Here's how the part is built. I have some questions about the finished solid (model axes, mm). Round coordinates to 2 decimals unless told otherwise and drop trailing zeros. Write each loop counter-clockwise with the first axis right and the second up, starting at its lowest first coordinate (ties: lowest second). Pieces come first, ordered by that corner, then holes. Notation, with made-up numbers: (38, -25.75) -> (79, -25.75) arc R34 ccw to (79, 11.25) -> close; hole circle Ø3 at (-18, 40.25). An arc over 180 degrees is marked (long way). Answer in a Markdown table with one row per item.
from build123d import *

# Parameters (mm, degrees)
SKETCH1_W           = 234.95
SKETCH1_H           = 228.6
BOSS_EXTRUDE1_DEPTH = 50.8
SKETCH2_R           = 4.826
CUT_EXTRUDE1_DEPTH  = 38.1
SKETCH3_R           = 6.477
CUT_EXTRUDE2_DEPTH  = 38.1


with BuildPart() as part:
    # Sketch1 → Boss-Extrude1 (new body)
    with BuildSketch(Plane(origin=(0, 0, 0), x_dir=(1, 0, 0), z_dir=(0, 1, 0))):
        with Locations((117.475, 114.3)):
            Rectangle(SKETCH1_W, SKETCH1_H)
    extrude(amount=BOSS_EXTRUDE1_DEPTH)

    # Sketch2 → Cut-Extrude1 (cut)
    with BuildSketch(Plane(origin=(0, 50.8, 0), x_dir=(1, 0, 0), z_dir=(0, 1, 0))):
        with Locations(Location((74.549, 170.307, 0), (0, 0, 270))):
            Circle(SKETCH2_R)
        with Locations(Location((160.401, 170.307, 0), (0, 0, 270))):
            Circle(SKETCH2_R)
        with Locations(Location((160.401, 58.293, 0), (0, 0, 270))):
            Circle(SKETCH2_R)
        with Locations(Location((74.549, 58.293, 0), (0, 0, 270))):
            Circle(SKETCH2_R)
    extrude(amount=-CUT_EXTRUDE1_DEPTH, mode=Mode.SUBTRACT)

    # Sketch3 → Cut-Extrude2 (cut)
    with BuildSketch(Plane(origin=(0, 50.8, 0), x_dir=(1, 0, 0), z_dir=(0, 1, 0))):
        with Locations(Location((196.85, 153.67, 0), (0, 0, 270))):
            Circle(SKETCH3_R)
        with Locations(Location((196.85, 74.93, 0), (0, 0, 270))):
            Circle(SKETCH3_R)
        with Locations(Location((38.1, 74.93, 0), (0, 0, 270))):
            Circle(SKETCH3_R)
        with Locations(Location((38.1, 153.67, 0), (0, 0, 270))):
            Circle(SKETCH3_R)
    extrude(amount=-CUT_EXTRUDE2_DEPTH, mode=Mode.SUBTRACT)


solid = part.part
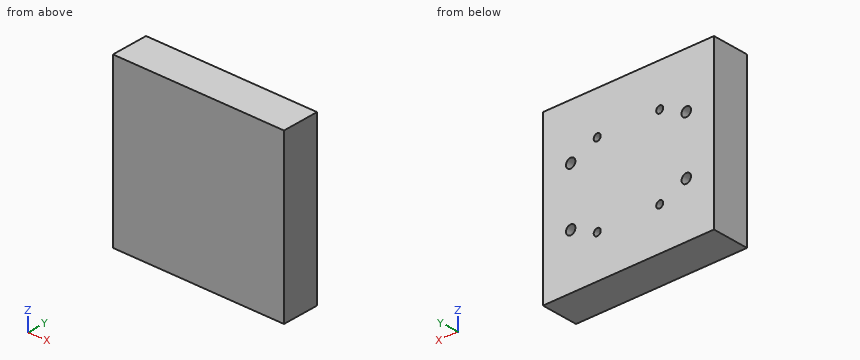
1) For pin 1 (4 mm diameter, centred on x = 38.5, z = -77, fed in from +Y), with a flat end and sliding along its axis, tell me the tip position at first contact or that it passes through.
Response:
| item | result |
|---|---|
| pin 1 | stops at y = 12.7 |
2) I need wall thicknesses on line 1 (X direction, y = 27.5, z = -74.93); line 2 (X direction, y = 22.5, z = -58.5). Which ranges of each line are inside material? Lowest first, please. Write a range as [from, to].
Response:
| item | result |
|---|---|
| line 1 | x = [0, 31.62], [44.58, 190.37], [203.33, 234.95] |
| line 2 | x = [0, 69.73], [79.37, 155.58], [165.22, 234.95] |
3) I want a section at C-C, the plane y = 22. Count the separate pieces of the cut face and the enclosed holes in it, and give its area (3 significant figures).
Response:
| item | result |
|---|---|
| separate pieces | 1 |
| enclosed holes | 8 |
| area | 52,900 mm^2 |
4) I want a section at B-B, the plane z = -153.67. List the corners of the cut face in (x, y) for me, and give its area (3 significant figures).
Response:
| item | result |
|---|---|
| outline | (0, 0) -> (234.95, 0) -> (234.95, 50.8) -> (203.33, 50.8) -> (203.33, 12.7) -> (190.37, 12.7) -> (190.37, 50.8) -> (44.58, 50.8) -> (44.58, 12.7) -> (31.62, 12.7) -> (31.62, 50.8) -> (0, 50.8) -> close |
| area | 10,900 mm^2 |
5) I want a section at A-A, the plane x = 38.1. List the corners of the cut face in (y, z) for me, and give its area (3 significant figures).
Response:
| item | result |
|---|---|
| outline | (0, -228.6) -> (50.8, -228.6) -> (50.8, -160.15) -> (12.7, -160.15) -> (12.7, -147.19) -> (50.8, -147.19) -> (50.8, -81.41) -> (12.7, -81.41) -> (12.7, -68.45) -> (50.8, -68.45) -> (50.8, 0) -> (0, 0) -> close |
| area | 10,600 mm^2 |
